Build history of the part. All positions in model axes, mm. A direction names the side the tool comes from. Coordinates: 2 decimals unless noted, no trailing zeros. Loops run counter-clockwise (first coordinate to the right, second up) from the corner with the lowest first, then second, coordinate; pieces in that order, holes last.
Item 1: 3-axis set-ups, long thin cutter, end or side, ignore diameter. For faces 5 (the face through (19.72, 1.384, -2.662)), 6 (the face through (39, -5, -3)), 7 (the face through (39, -5, 3)): which of +Z, -Z, +X, -X, +Y, -Y reach the whole face in a straight line?
Item 2: Drill centre lines: line 1 along Z through (x, y) = (1.25, 0); line 2 along Z through (x, y) = (16.5, 0); line 3 along X through (y, z) = (-7.5, -1.5). Where is each one in solid material? Low to high.
Item 3: Cut at D-D (x = 29.5). List the corners of the cut face in (y, z).
Item 4: Cut at B-B (z = 0.5). List the corners of the cut face in (x, y).
Item 5: Cut at A-A (x = 37.5). List the corners of the cut face in (y, z), and give its area (3 significant figures).
Item 6: Flat gauge pins, fed straight in: pin 1 (3 mm diameter, centred on y = -1, z = 8, fed in from +X); pin 2 (6.5 mm diameter, centred on y = -9, z = -0.5, fed in from -X); pin 3 (8 mm diameter, centred on x = 16, z = 4, fed in from +Y); pin 4 (5 mm diameter, centred on x = 16.5, y = -4.5, fed in from +Z). Where does each tip first touch, or does it go through?
Item 7: Mould opens along Y. For faces 1 (the face through (1, -3, 5)), 2 (the face through (37, -7, 0)), 3 (the face through (1, 3, 5)), 4 (the face through (1, 0, 11)) say: released by +Y, released by -Y, zero draft, split by the parting line, or undercut.
Item 8: Cut at C-C (y = -2). List the corners of the cut face in (x, z).
from build123d import *

# Parameters (mm, degrees)
F0_R     = 3
F0_R_2   = 1.5
F1_DEPTH = 40
F3_DEPTH = 3
F5_DEPTH = 3


with BuildPart() as f1:
    # F0 (on Right) → F1 (new body)
    with BuildSketch(Plane.YZ):
        Circle(F0_R)
        Circle(F0_R_2, mode=Mode.SUBTRACT)
    extrude(amount=F1_DEPTH)

    # F2 (on face) → F3 (join)
    with BuildSketch(Plane.YZ.offset(40)):
        with BuildLine():
            Line((-10, -3), (0, -3))
            ThreePointArc((0, -3), (-3, 0), (0, 3))
            Line((0, 3), (-10, 3))
            ThreePointArc((-10, 3), (-7.8786796564, 2.1213203436), (-7, 0))
            ThreePointArc((-7, 0), (-7.8786796564, -2.1213203436), (-10, -3))
        make_face()
        with BuildLine():
            Line((-10, -1), (-10, -3))
            ThreePointArc((-10, -3), (-7.8786796564, -2.1213203436), (-7, 0))
            ThreePointArc((-7, 0), (-7.8786796564, 2.1213203436), (-10, 3))
            Line((-10, 3), (-10, 1))
            ThreePointArc((-10, 1), (-9.2928932188, 0.7071067812), (-9, 0))
            ThreePointArc((-9, 0), (-9.2928932188, -0.7071067812), (-10, -1))
        make_face()
        with BuildLine():
            ThreePointArc((-10, 3), (-13, 0), (-10, -3))
            Line((-10, -3), (-10, -1))
            ThreePointArc((-10, -1), (-11, 0), (-10, 1))
            Line((-10, 1), (-10, 3))
        make_face()
    extrude(amount=-F3_DEPTH)

    # F4 (on face) → F5 (join)
    with BuildSketch(Plane(origin=(0, 0, 0), x_dir=(0, -1, 0), z_dir=(-1, 0, 0))):
        with BuildLine():
            ThreePointArc((-3, 0), (0, 3), (3, 0))
            Line((3, 0), (3, 10))
            ThreePointArc((3, 10), (0, 7), (-3, 10))
            Line((-3, 10), (-3, 0))
        make_face()
        with BuildLine():
            ThreePointArc((-3, 10), (0, 7), (3, 10))
            Line((3, 10), (1, 10))
            ThreePointArc((1, 10), (0, 9), (-1, 10))
            Line((-1, 10), (-3, 10))
        make_face()
        with BuildLine():
            Line((1, 10), (3, 10))
            ThreePointArc((3, 10), (0, 13), (-3, 10))
            Line((-3, 10), (-1, 10))
            ThreePointArc((-1, 10), (0, 11), (1, 10))
        make_face()
    extrude(amount=-F5_DEPTH)


solid = f1.part
Filled sheet:
1. face 5: none
1. face 6: -Z, +X, -X, +Y, -Y
1. face 7: +Z, +X, +Y, -Y
2. line 1: z = -3 to -1.5, 1.5 to 9, 11 to 13
2. line 2: z = -3 to -1.5, 1.5 to 3
2. line 3: x = 37 to 40
3. outline: circle Ø6 at (0, 0); hole circle Ø3 at (0, 0)
4. outline: (0, -3) - (3, -3) - (3, -2.96) - (37, -2.96) - (37, -9.13) - (40, -9.13) - (40, -1.41) - (0, -1.41) - close; (0, 1.41) - (40, 1.41) - (40, 2.96) - (3, 2.96) - (3, 3) - (0, 3) - close; (37, -12.96) - (40, -12.96) - (40, -10.87) - (37, -10.87) - close
5. outline: (-10, -3) - (0, -3) arc R3 ccw to (0, 3) - (-10, 3) arc R3 ccw to start; hole circle Ø2 at (-10, 0); hole circle Ø3 at (0, 0)
5. area: 78.1 mm2
6. pin 1: stops at x = 3
6. pin 2: stops at x = 37
6. pin 3: stops at y = 3
6. pin 4: stops at z = 2.24
7. face 1: released by -Y
7. face 2: zero draft
7. face 3: released by +Y
7. face 4: undercut
8. outline: (0, -2.24) - (37, -2.24) - (37, -3) - (40, -3) - (40, 3) - (37, 3) - (37, 2.24) - (3, 2.24) - (3, 12.24) - (0, 12.24) - close
